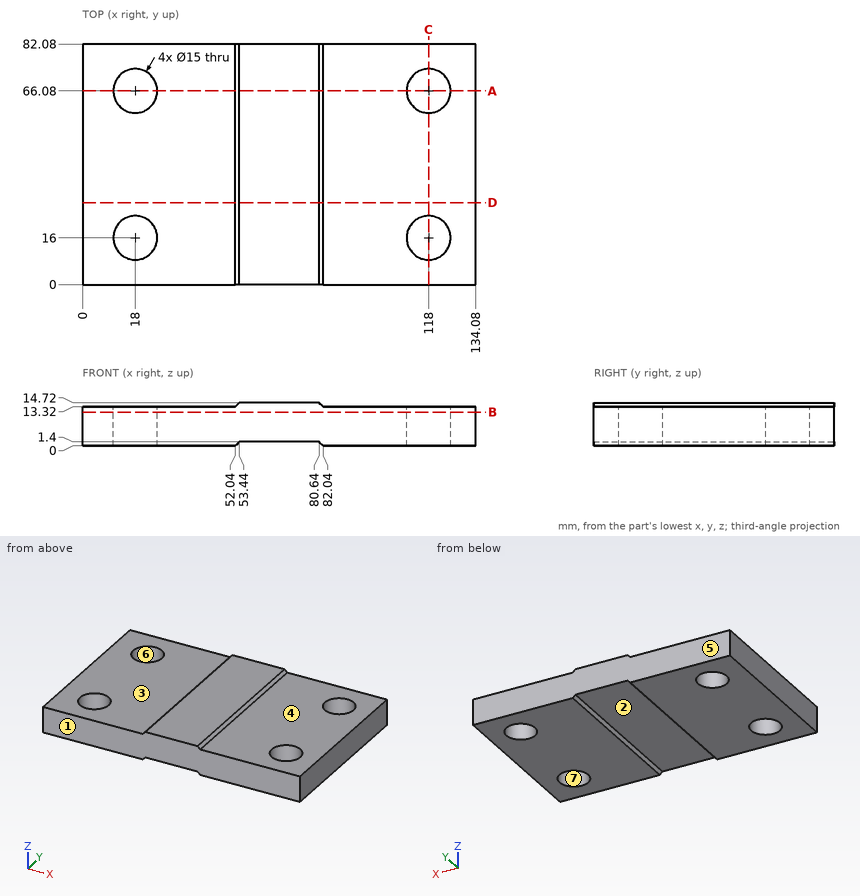
Source: three-view drawing plus pictorial views. Frame: mm from the lowest corner of the part. A direction names the side the tool comes from. Coordinates: 2 decimals unless noted, no trailing zeros. Loops run counter-clockwise (first coordinate to the right, second up) from the corner with the lowest first, then second, coordinate; pieces in that order, holes last. Notation, with made-up numbers: (34.25, 67.5) - (75.25, 67.5) arc R18 ccw to (75.25, 80.5) - close; hole circle Ø4 at (-38.5, 80). An arc over 180 degrees is marked (long way). One line per item, written item: value. Start each with the question number.
1. Section C-C (x = 118). Return the cut outline in (y, z), and give its area (3 significant figures).
2. Ray query, L1, parallel to Y at x = 118, z = 5.5; L2, parallel to X at y = 66.08, z = 6.5; L3, parallel to X at y = 13.5, z = 9.75. Return the intervals inside material, ascending.
3. Set-up query: the marked faces 1, 2 and 3. Return all of +Z, -Z, +X, -X, +Y, -Y with unobstructed straight access to the full face (end or side cutting, diameter ignored); none if empty.
4. Section A-A (y = 66.08). Return the cut outline in (x, z), and give its area (3 significant figures).
5. Mould query, pull axis Y, two halves, no side actions, for the marked faces 4, 5, 6 and 7. Classes: pulls with the +Y half, pulls with the -Y half, needs draft (parallel to the pull), parting line crosses it, or undercut.
6. Section B-B (z = 11.5). Return the cut outline in (x, y), and give its area (3 significant figures).
7. Section D-D (y = 28). Return the cut outline in (x, z).
8. Contact query for flat-ended pins moving along their axis: P1, Ø1.5, axis at x = 24.5, y = 39.5, coming from the +Z side; P2, Ø22, axis at x = 68, y = 60.5, coming from the -Z side. Output: stop coordinate, or through.
Verdict:
1. outline: (0, 0) - (8.5, 0) - (8.5, 13.32) - (0, 13.32) - close; (23.5, 0) - (58.58, 0) - (58.58, 13.32) - (23.5, 13.32) - close; (73.58, 0) - (82.08, 0) - (82.08, 13.32) - (73.58, 13.32) - close
1. area: 694 mm2
2. L1: y = 0 to 8.5, 23.5 to 58.58, 73.58 to 82.08
2. L2: x = 0 to 10.5, 25.5 to 110.5, 125.5 to 134.08
2. L3: x = 0 to 10.93, 25.07 to 110.93, 125.07 to 134.08
3. face 1: +Z, -Z, +X, -X, -Y
3. face 2: -Z, +Y, -Y
3. face 3: +Z, -X, +Y, -Y
4. outline: (0, 0) - (10.5, 0) - (10.5, 13.32) - (0, 13.32) - close; (25.5, 0) - (52.04, 0) - (53.44, 1.4) - (80.64, 1.4) - (82.04, 0) - (110.5, 0) - (110.5, 13.32) - (82.04, 13.32) - (80.64, 14.72) - (53.44, 14.72) - (52.04, 13.32) - (25.5, 13.32) - close; (125.5, 0) - (134.08, 0) - (134.08, 13.32) - (125.5, 13.32) - close
4. area: 1,390 mm2
5. face 4: needs draft
5. face 5: pulls with the +Y half
5. face 6: undercut
5. face 7: undercut
6. outline: (0, 0) - (134.08, 0) - (134.08, 82.08) - (0, 82.08) - close; hole circle Ø15 at (18, 16); hole circle Ø15 at (18, 66.08); hole circle Ø15 at (118, 16); hole circle Ø15 at (118, 66.08)
6. area: 10,300 mm2
7. outline: (0, 0) - (52.04, 0) - (53.44, 1.4) - (80.64, 1.4) - (82.04, 0) - (134.08, 0) - (134.08, 13.32) - (82.04, 13.32) - (80.64, 14.72) - (53.44, 14.72) - (52.04, 13.32) - (0, 13.32) - close
8. P1: stops at z = 13.32
8. P2: stops at z = 1.4
